Design review of the part built by this model. Coordinates are the model's own, in mm. A direction names the side the tool comes from. Coordinates: 2 decimals unless noted, no trailing zeros. Loops run counter-clockwise (first coordinate to the right, second up) from the corner with the lowest first, then second, coordinate; pieces in that order, holes last.
Autodesk Inventor part; units mm, degrees
ref_plane "YZ Plane" through (0, 0, 0) normal (1, 0, 0) x (0, 1, 0)
ref_plane "XZ Plane" through (0, 0, 0) normal (0, 1, 0) x (-1, 0, 0)
ref_plane "XY Plane" through (0, 0, 0) normal (0, 0, 1) x (1, 0, 0)
sketch "Sketch8" plane through (0, 0, 0) normal (0, 0, 1) x (1, 0, 0)
  line L0 (0, 0) -> (41, 0)
  line L1 (41, 0) -> (41, 21)
  line L2 (41, 21) -> (0, 21)
  line L3 (0, 21) -> (0, 0)
  line L4 (-6, 27) -> (47, 27)
  line L5 (47, 27) -> (47, -6)
  line L6 (47, -6) -> (-6, -6)
  line L7 (-6, -6) -> (-6, 27)
  dimension "d35" = 41
  dimension "d36" = 21
  dimension "d37" = 6
extrude "Extrusion8" add sketch "Sketch8" along normal blind 20
sketch "Sketch9" plane through (0, 0, 20) normal (0, 0, 1) x (1, 0, 0)
  line L0 (41, 0) -> (0, 0)
  line L1 (20.5, 0) -> (10.5, 0)
  line L2 (10.5, 0) -> (10.5, -5)
  line L3 (10.5, -5) -> (30.5, -5)
  line L4 (30.5, -5) -> (30.5, 0)
  line L5 (30.5, 0) -> (20.5, 0)
  dimension "d45" = 10
  dimension "d46" = 5
  dimension "d47" = 20
  dimension "d48" = 5
extrude "Extrusion9" cut sketch "Sketch9" against normal up to next
sketch "Sketch10" plane through (0, 0, 20) normal (0, 0, 1) x (1, 0, 0)
  line L0 (0, 21) -> (0, 0)
  line L1 (0, 10.5) -> (41, 10.5)
  line L2 (41, 21) -> (41, 0)
  circle A0 centre (20.5, 10.5) radius 20
  circle A1 centre (20.5, 10.5) radius 26.5
  line L3 (47, 27) -> (47, -6)
  dimension "d51" = 40
extrude "Extrusion10" add sketch "Sketch10" along normal blind 13
equation "\"BendRadius\" = Thickness"
equation "\"BendReliefWidth\" = Thickness"
equation "\"BendReliefDepth\" = 0.5 * Thickness"
equation "\"CornerReliefSize\" = 4 * Thickness"
equation "\"MinimumRemnant\" = 2 * Thickness"
equation "\"TransitionRadius\" = BendRadius"
equation "\"JacobiRadiusSize\" = BendRadius"
equation "\"GapSize\" = Thickness"
properties part number "baseRotor1"
Q1. For line 1 (Y direction, x = 21, z = 24.5); line 2 (Y direction, x = 7.5, z = 2); line 3 (X direction, y = 12.5, z = 17), list the stretches that pass through material, from the lowest coordinate up.
Q2. Take a section at D-D, the plane x = 7.5. Write out the cut boundary in (y, z).
Q3. The part is to be moulded in two halves that separate along X. For faces 6 (the flat face through (10.5, -2, 10)), 7 (the flat face through (20, 22, 0)), 8 (the flat face through (47, 11, 10)), say which applies: pulls with the +X half, pulls with the -X half, needs draft (parallel to the pull), parting line crosses it, or undercut.
Q4. Take a section at A-A, the plane x = 20.5. Write out the cut boundary in (y, z), then the cut area to 3 significant figures.
Q5. Clearance check with flat-ended pins moving along their axes: pin 1 Ø5 at (x, y) = (14.5, -9.5) entering from -Z; pin 2 Ø5 at (x, z) = (5, 12.5) entering from +Y; pin 3 Ø3 at (x, z) = (40, 16) entering from -Y. State where each tip first meets the part, or that it passes through.
Q6. Take a section at B-B, the plane z = 2.5. Write out the cut boundary in (x, y).
Q7. Take a section at C-C, the plane y = 29. Write out the cut boundary in (x, z).
Q8. Machinability: for faces 1 (the flat face through (41, 10, 10)), 2 (the flat face through (20, 32, 20)), 3 (the flat face through (45, 22, 20)), 4 (the flat face through (20, 24, 20)), 5 (the flat face through (-4, -2, 20)), which of the approach directions +Z, -Z, +X, -X, +Y, -Y give a long, thin tool a straight path to every point of the face, cutting with its end or side? Answer none if there is none.
Entries:
1. line 1: y = -16 to -9.49, 30.49 to 37
1. line 2: y = -6 to 0, 21 to 27
1. line 3: x = -6 to 0, 41 to 47
2. outline: (-12.59, 20) - (-6, 20) - (-6, 0) - (0, 0) - (0, 20) - (-4.7, 20) - (-4.7, 33) - (-12.59, 33) - close; (21, 0) - (27, 0) - (27, 20) - (33.59, 20) - (33.59, 33) - (25.7, 33) - (25.7, 20) - (21, 20) - close
3. face 6: undercut
3. face 7: needs draft
3. face 8: pulls with the +X half
4. outline: (-16, 20) - (-9.5, 20) - (-9.5, 33) - (-16, 33) - close; (-6, 0) - (-5, 0) - (-5, 20) - (-6, 20) - close; (21, 0) - (27, 0) - (27, 20) - (21, 20) - close; (30.5, 20) - (37, 20) - (37, 33) - (30.5, 33) - close
4. area: 309 mm2
5. pin 1: stops at z = 20
5. pin 2: stops at y = 27
5. pin 3: stops at y = -6
6. outline: (-6, -6) - (47, -6) - (47, 27) - (-6, 27) - close; hole (0, 0) - (10.5, 0) - (10.5, -5) - (30.5, -5) - (30.5, 0) - (41, 0) - (41, 21) - (0, 21) - close
7. outline: (1.53, 20) - (12.9, 20) - (12.9, 33) - (1.53, 33) - close; (28.1, 20) - (39.47, 20) - (39.47, 33) - (28.1, 33) - close
8. face 1: -Z
8. face 2: -Z, +X, -X, +Y
8. face 3: +Z, +X, +Y
8. face 4: +Z
8. face 5: +Z, -X, -Y
